Work out the finished part from the listing and answer in its coordinate system (mm). Coordinates: 2 decimals unless noted, no trailing zeros. Order: outer loops, then holes, each group sorted by start corner. A loop starts at its lowest first (then second) coordinate and runs counter-clockwise, first axis right, second up. Notation, with made-up numbers: (-9, 68.5) -> (38, 68.5) arc R9 ccw to (38, 80.5) -> close; hole circle Ø9 at (81.25, -15.5). An arc over 180 degrees is marked (long way). Write item = value, one per line. Start each with the question number.
Q1. Flat-ended cylindrical pins translate along their axes: pin 1 (0.5 mm diameter, centred on y = -7, z = 0, fed in from +X); pin 2 (0.8 mm diameter, centred on x = 0, z = 0, fed in from +Y); pin 3 (0.5 mm diameter, centred on x = 10, y = -5.5, fed in from -Z). Find the tip coordinate at first contact, or state that the pin passes through.
Q2. Straight lines are drawn through the part: L1, parallel to X at y = -4, z = -0.1; L2, parallel to Y at x = 13.25, z = 0.3; L3, parallel to Z at x = 10, y = -8. For each, find the intervals that lie inside material, in ascending order. Write a range as from..to.
Q3. The part is cut by section D-D, the plane x = 12. Determine the outline of the cut face in (y, z) (3 decimals), plus the area to 3 significant figures.
Q4. The part is cut by section C-C, the plane y = -1.25. Determine the outline of the cut face in (x, z).
Q5. For a pull along X with two mould halves and no side action, classify faces 1 (the flat face through (-1.27, 4, 0)), 2 (the flat face through (13, 6, 0.5)), 3 (the flat face through (7.12, 6, 0)), 4 (the flat face through (6, 4, 1.205)) as +X half, -X half, draft (parallel to the pull), parting line (faces both ways), or undercut.
Q6. The part is cut by section A-A, the plane y = 4.5. Determine the outline of the cut face in (x, z) (3 decimals).
Q7. The part is cut by section B-B, the plane z = -0.8. Determine the outline of the cut face in (x, y).
```python
from build123d import *

# Parameters (mm, degrees)
SKETCH2_W                  = 15.24
SKETCH2_H                  = 2.41
BOSS_EXTRUDE1_DEPTH        = 8.51
SKETCH5_W                  = 1
SKETCH5_H                  = 1
CUT_EXTRUDE1_DEPTH         = 5
CHAMFER1_SIZE              = 0.5
LPATTERN3_COUNT            = 6
LPATTERN3_PITCH            = 2.54
CHAMFER1_OF_LPATTERN3_SIZE = 0.5
SKETCH11_W                 = 0.64
SKETCH11_H                 = 0.64
BOSS_EXTRUDE2_DEPTH        = 9.92
LPATTERN4_COUNT            = 6
LPATTERN4_PITCH            = 2.54


with BuildPart() as part:
    # Sketch2 → Boss-Extrude1 (new body)
    with BuildSketch(Plane(origin=(0, 0, 0), x_dir=(1, 0, 0), z_dir=(0, 1, 0))):
        with Locations((6.35, 0)):
            Rectangle(SKETCH2_W, SKETCH2_H)
    extrude(amount=BOSS_EXTRUDE1_DEPTH)

    # Sketch5 → Cut-Extrude1 (cut)
    with BuildSketch(Plane(origin=(0, 8.51, 0), x_dir=(1, 0, 0), z_dir=(0, 1, 0))):
        Rectangle(SKETCH5_W, SKETCH5_H)
    cut_extrude1 = extrude(amount=-CUT_EXTRUDE1_DEPTH, mode=Mode.SUBTRACT)

    # Chamfer1
    chamfer1_edges = [part.edges().sort_by_distance(p)[0] for p in [
        (0.5, 8.51, 0),
        (0, 8.51, -0.5),
        (-0.5, 8.51, 0),
        (0, 8.51, 0.5),
    ]]
    chamfer(chamfer1_edges, length=CHAMFER1_SIZE)

    # LPattern3: Cut-Extrude1 ×6
    with Locations(*[(i * LPATTERN3_PITCH, 0, 0) for i in range(1, LPATTERN3_COUNT)]):
        add(cut_extrude1, mode=Mode.SUBTRACT)

    # Chamfer1 of LPattern3
    chamfer1_of_lpattern3_edges = [part.edges().sort_by_distance(p)[0] for p in [
        (3.04, 8.51, 0),
        (2.54, 8.51, -0.5),
        (2.04, 8.51, 0),
        (2.54, 8.51, 0.5),
        (5.58, 8.51, 0),
        (5.08, 8.51, -0.5),
        (4.58, 8.51, 0),
        (5.08, 8.51, 0.5),
        (8.12, 8.51, 0),
        (7.62, 8.51, -0.5),
        (7.12, 8.51, 0),
        (7.62, 8.51, 0.5),
        (10.66, 8.51, 0),
        (10.16, 8.51, -0.5),
        (9.66, 8.51, 0),
        (10.16, 8.51, 0.5),
        (13.2, 8.51, 0),
        (12.7, 8.51, -0.5),
        (12.2, 8.51, 0),
        (12.7, 8.51, 0.5),
    ]]
    chamfer(chamfer1_of_lpattern3_edges, length=CHAMFER1_OF_LPATTERN3_SIZE)

    # Sketch11 → Boss-Extrude2 (add)
    with BuildSketch(Plane.XZ):
        Rectangle(SKETCH11_W, SKETCH11_H)
    boss_extrude2 = extrude(amount=BOSS_EXTRUDE2_DEPTH)

    # Sketch13 → Loft1 section 0
    with BuildSketch(Plane.XZ.offset(9.92)):
        with BuildLine():
            Line((0.32, -0.32), (0.32, 0.32))
            Line((0.32, 0.32), (-0.32, 0.32))
            Line((-0.32, 0.32), (-0.32, -0.32))
            Line((-0.32, -0.32), (0.32, -0.32))
        make_face()
    # Sketch14 → Loft1 section 1
    with BuildSketch(Plane(origin=(0, -10.49, 0), x_dir=(-1, 0, 0), z_dir=(0, -1, 0))):
        with BuildLine():
            Line((-0.22, 0.22), (0.22, 0.22))
            Line((0.22, 0.22), (0.22, -0.22))
            Line((0.22, -0.22), (-0.22, -0.22))
            Line((-0.22, -0.22), (-0.22, 0.22))
        make_face()
    loft1 = loft()

    # LPattern4: Boss-Extrude2, Loft1 ×6
    with Locations(*[(i * LPATTERN4_PITCH, 0, 0) for i in range(1, LPATTERN4_COUNT)]):
        add(boss_extrude2)
        add(loft1)


solid = part.part
```
Model answer:
q1.pin_1 = 13.02
q1.pin_2 = 3.51
q1.pin_3 = -0.32
q2.L1 = -0.32..0.32, 2.22..2.86, 4.76..5.4, 7.3..7.94, 9.84..10.48, 12.38..13.02
q2.L2 = 0..8.06
q2.L3 = -0.32..0.32
q3.outline = (0, -1.205) -> (8.51, -1.205) -> (8.51, -1) -> (8.21, -0.7) -> (8.21, 0.7) -> (8.51, 1) -> (8.51, 1.205) -> (0, 1.205) -> close
q3.area = 20.0 mm2
q4.outline = (-0.32, -0.32) -> (0.32, -0.32) -> (0.32, 0.32) -> (-0.32, 0.32) -> close; (2.22, -0.32) -> (2.86, -0.32) -> (2.86, 0.32) -> (2.22, 0.32) -> close; (4.76, -0.32) -> (5.4, -0.32) -> (5.4, 0.32) -> (4.76, 0.32) -> close; (7.3, -0.32) -> (7.94, -0.32) -> (7.94, 0.32) -> (7.3, 0.32) -> close; (9.84, -0.32) -> (10.48, -0.32) -> (10.48, 0.32) -> (9.84, 0.32) -> close; (12.38, -0.32) -> (13.02, -0.32) -> (13.02, 0.32) -> (12.38, 0.32) -> close
q5.face_1 = -X half
q5.face_2 = undercut
q5.face_3 = undercut
q5.face_4 = draft
q6.outline = (-1.27, -1.205) -> (13.97, -1.205) -> (13.97, 1.205) -> (-1.27, 1.205) -> close; hole (-0.5, -0.5) -> (0.5, -0.5) -> (0.5, 0.5) -> (-0.5, 0.5) -> close; hole (2.04, -0.5) -> (3.04, -0.5) -> (3.04, 0.5) -> (2.04, 0.5) -> close; hole (4.58, -0.5) -> (5.58, -0.5) -> (5.58, 0.5) -> (4.58, 0.5) -> close; hole (7.12, -0.5) -> (8.12, -0.5) -> (8.12, 0.5) -> (7.12, 0.5) -> close; hole (9.66, -0.5) -> (10.66, -0.5) -> (10.66, 0.5) -> (9.66, 0.5) -> close; hole (12.2, -0.5) -> (13.2, -0.5) -> (13.2, 0.5) -> (12.2, 0.5) -> close
q7.outline = (-1.27, 0) -> (13.97, 0) -> (13.97, 8.51) -> (13.7, 8.51) -> (13.5, 8.31) -> (11.9, 8.31) -> (11.7, 8.51) -> (11.16, 8.51) -> (10.96, 8.31) -> (9.36, 8.31) -> (9.16, 8.51) -> (8.62, 8.51) -> (8.42, 8.31) -> (6.82, 8.31) -> (6.62, 8.51) -> (6.08, 8.51) -> (5.88, 8.31) -> (4.28, 8.31) -> (4.08, 8.51) -> (3.54, 8.51) -> (3.34, 8.31) -> (1.74, 8.31) -> (1.54, 8.51) -> (1, 8.51) -> (0.8, 8.31) -> (-0.8, 8.31) -> (-1, 8.51) -> (-1.27, 8.51) -> close
